CAD build for the part. Positions are in the model's coordinates, mm. A direction names the side the tool comes from. Give positions to 0.01 mm unless a question says otherwise; leave off trailing zeros. Order: outer loops, then holes, each group sorted by start corner. A loop starts at its lowest first (then second) coordinate and runs counter-clockwise, first axis right, second up.
Item 1: Wall check: L1, parallel to X at y = 0, z = 20.5; L2, parallel to X at y = 29.5, z = -1.5; L3, parallel to Y at x = -3.5, z = 10. Give the ranges that are in metal, low to high.
Item 2: Band-saw the part on B-B on z = -8.5. Give the cut face in (x, y), plus the area to 3 significant figures.
Item 3: Band-saw the part on C-C on z = 12.5. Give the cut face in (x, y), plus the area to 4 significant figures.
Item 4: Which spindle directions (+Z, -Z, +X, -X, +Y, -Y) get a long thin tool onto all of the face, cutting with end or side? Do faces 1 (the flat face through (-21.75, 31, -1)), 2 (the flat face through (-6.75, 28, -7)), 3 (the flat face through (26.75, 28, -7)), 4 (the flat face through (11.75, 31, -1)), 5 (the flat face through (-17, 25.171, -11)). Say none if no direction does.
Item 5: Band-saw the part on D-D on y = 21. Give the cut face in (x, z).
Item 6: Flat gauge pins, fed straight in: P1, Ø1.5, axis at y = 29, z = -6.5, coming from the -X side; P2, Ø10, axis at x = -11, z = 10.5, coming from the +Y side; P3, Ø16.5, axis at x = -15.5, z = -4, coming from the -Y side; P4, Ø4, axis at x = -17.5, y = 26.5, coming from the +Z side. Where does each tip first touch, or does it go through?
Item 7: Band-saw the part on A-A on x = 13. Give the cut face in (y, z), plus the area to 3 significant figures.
Item 8: Two-plate mould, pull along Z, no slides. Class faces 6 (the flat face through (0, 8, 1.5)), 7 (the flat face through (17, 28, -15)), 8 (the flat face through (-17, 26.921, -2)), 9 (the flat face through (32, 8, 12)): released by +Z, released by -Z, zero draft, split by the parting line, or undercut.
```python
from build123d import *

# Parameters (mm, degrees)
F0_W      = 64
F0_H      = 1.5
F1_DEPTH  = 23
F0_H_2    = 83
F2_DEPTH  = 1.5
F5_W      = 10
F5_H      = 1.5
F6_DEPTH  = 4.5
F7_W      = 10
F7_H      = 4.5
F9_DEPTH  = 5
F11_DEPTH = 50
F12_DEPTH = 10
F13_W     = 5
F13_H     = 5
F14_DEPTH = 53.5
F15_W     = 13.5
F15_H     = 5
F16_DEPTH = 25


with BuildPart() as f1:
    # F0 (on Top) → F1 (new body)
    with BuildSketch(Plane.XY):
        Polygon((-32, 48.42079), (-33.5, 48.42079), (-33.5, -36.07921), (-32, -36.07921), (-32, -34.57921), align=None)
        with Locations((0, -35.32921)):
            Rectangle(F0_W, F0_H)
        Polygon((33.5, 48.42079), (32, 48.42079), (32, -34.57921), (32, -36.07921), (33.5, -36.07921), align=None)
    extrude(amount=F1_DEPTH)

    # F0 (on Top) → F2 (join)
    with BuildSketch(Plane.XY):
        Polygon((-32, 48.42079), (-33.5, 48.42079), (-33.5, -36.07921), (-32, -36.07921), (-32, -34.57921), align=None)
        with Locations((0, 6.92079)):
            Rectangle(F0_W, F0_H_2)
        Polygon((33.5, 48.42079), (32, 48.42079), (32, -34.57921), (32, -36.07921), (33.5, -36.07921), align=None)
        with Locations((0, -35.32921)):
            Rectangle(F0_W, F0_H)
    extrude(amount=F2_DEPTH)


with BuildPart() as f3_1:
    # F3: copy of F1
    add(f1.part)

    # F5 (on face) → F6 (join)
    with BuildSketch(Plane(origin=(0, 0, 0), x_dir=(1, 0, 0), z_dir=(0, 0, -1))):
        with Locations((16.75, -27.67079)):
            Rectangle(F5_W, F5_H)
        with Locations((-16.75, -27.67079)):
            Rectangle(F5_W, F5_H)
    extrude(amount=F6_DEPTH)

    # F7 (on face) → F9 (join)
    with BuildSketch(Plane(origin=(0, 28.42079, 0), x_dir=(-1, 0, 0), z_dir=(0, 1, 0))):
        with Locations((-16.75, -2.25)):
            Rectangle(F7_W, F7_H)
        with Locations((16.75, -2.25)):
            Rectangle(F7_W, F7_H)
    extrude(amount=F9_DEPTH)

    # F10 (on face) → F11 (cut)
    with BuildSketch(Plane.YZ.offset(21.75)):
        Polygon((33.42079, -4.5), (33.42079, 0), (26.92079, -4.5), align=None)
    extrude(amount=-F11_DEPTH, mode=Mode.SUBTRACT)

    # F8 (on face) → F12 (join)
    with BuildSketch(Plane(origin=(0, 0, 0), x_dir=(1, 0, 0), z_dir=(0, 0, -1))):
        Polygon((-21.75, -26.92079), (-21.75, -25.17079), (-26.75, -25.17079), (-26.75, -30.17079), (-21.75, -30.17079), (-21.75, -28.42079), align=None)
        Polygon((-11.75, -25.17079), (-11.75, -26.92079), (-11.75, -28.42079), (-11.75, -30.17079), (-6.75, -30.17079), (-6.75, -25.17079), align=None)
        Polygon((11.75, -25.17079), (6.75, -25.17079), (6.75, -30.17079), (11.75, -30.17079), (11.75, -28.42079), (11.75, -26.92079), align=None)
        Polygon((21.75, -25.17079), (21.75, -26.92079), (21.75, -28.42079), (21.75, -30.17079), (26.75, -30.17079), (26.75, -25.17079), align=None)
    extrude(amount=F12_DEPTH)

    # F13 (on face) → F14 (join)
    with BuildSketch(Plane.YZ.offset(26.75)):
        with Locations((27.67079, -12.5)):
            Rectangle(F13_W, F13_H)
    extrude(amount=-F14_DEPTH)

    # F15 (on face) → F16 (cut)
    with BuildSketch(Plane(origin=(0, 30.17079, 0), x_dir=(-1, 0, 0), z_dir=(0, 1, 0))):
        with Locations((0, -12.5)):
            Rectangle(F15_W, F15_H)
    extrude(amount=-F16_DEPTH, mode=Mode.SUBTRACT)


solid = f3_1.part
```
The answers:
1. L1: x = -33.5 to -32, 32 to 33.5
1. L2: x = -26.75 to -6.75, 6.75 to 26.75
1. L3: y = -36.08 to -34.58
2. outline: (-26.75, 25.17) - (-21.75, 25.17) - (-21.75, 30.17) - (-26.75, 30.17) - close; (-11.75, 25.17) - (-6.75, 25.17) - (-6.75, 30.17) - (-11.75, 30.17) - close; (6.75, 25.17) - (11.75, 25.17) - (11.75, 30.17) - (6.75, 30.17) - close; (21.75, 25.17) - (26.75, 25.17) - (26.75, 30.17) - (21.75, 30.17) - close
2. area: 100 mm2
3. outline: (-33.5, -36.08) - (33.5, -36.08) - (33.5, 48.42) - (32, 48.42) - (32, -34.58) - (-32, -34.58) - (-32, 48.42) - (-33.5, 48.42) - close
3. area: 349.5 mm2
4. face 1: -Z, -X, +Y
4. face 2: -Z, +Y, -Y
4. face 3: -Z, +X, +Y, -Y
4. face 4: -Z, +Y
4. face 5: -Z, +X, -X, -Y
5. outline: (-33.5, 0) - (33.5, 0) - (33.5, 23) - (32, 23) - (32, 1.5) - (-32, 1.5) - (-32, 23) - (-33.5, 23) - close
6. P1: stops at x = -26.75
6. P2: stops at y = -34.58
6. P3: stops at y = -36.08
6. P4: stops at z = 1.5
7. outline: (-36.08, 0) - (26.92, 0) - (26.92, -4.5) - (33.42, 0) - (48.42, 0) - (48.42, 1.5) - (-34.58, 1.5) - (-34.58, 23) - (-36.08, 23) - close; (25.17, -15) - (30.17, -15) - (30.17, -10) - (25.17, -10) - close
7. area: 199 mm2
8. face 6: released by +Z
8. face 7: released by -Z
8. face 8: undercut
8. face 9: zero draft
